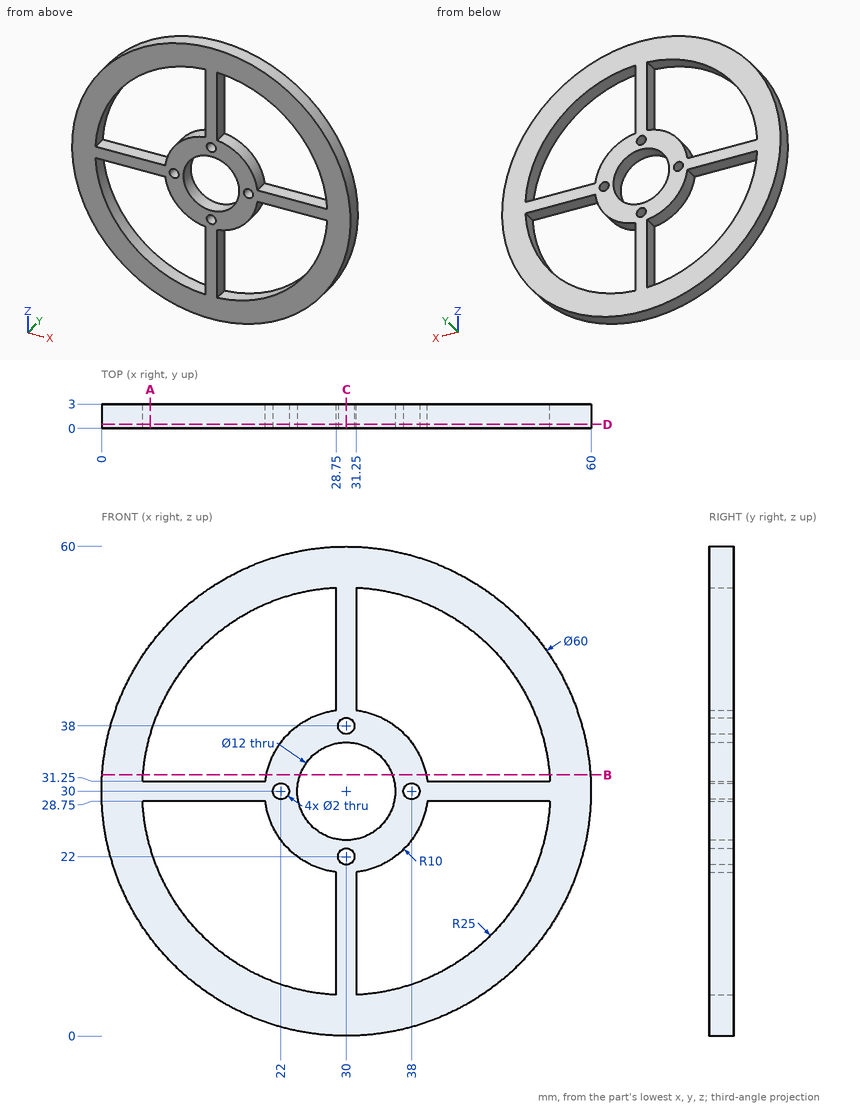
For this review, use the dimensioned drawing (mm, ordinates from the lowest corner) and the shaded views. Give positions to 0.01 mm unless a question says otherwise; leave off trailing zeros. Order: outer loops, then holes, each group sorted by start corner. A loop starts at its lowest first (then second) coordinate and runs counter-clockwise, first axis right, second up.
1) Wall thickness on line 1 (X direction, y = 2.35, z = 30); line 2 (Z direction, x = 36.5, y = 0.6); line 3 (Z direction, x = 49.5, y = 1.95): over which ranges is each line inside the solid? List them lowest first.
2) Take a section at A-A (x = 6). Give the boundary of the cut face in (y, z).
3) Insertion check: pin 1 (1 mm diameter, centred on x = 39, y = 2, fed in from -Z); pin 2 (1.5 mm diameter, centred on x = 13, y = 2, fed in from -Z); pin 3 (1.5 mm diameter, centred on y = 1.5, z = 40.5, fed in from +X). Each pin has a flat end and moves straight along its axis. Give the tip position at first contact, or say it passes through.
4) Take a section at B-B (z = 32). Give the boundary of the cut face in (x, y).
5) Take a section at C-C (x = 30). Give the boundary of the cut face in (y, z).
6) Take a section at D-D (y = 0.5). State how many separate pieces and enclosed holes the cut face has, then the cut area to 3 significant figures.
Derived:
1. line 1: x = 0 to 21, 23 to 24, 36 to 37, 39 to 60
1. line 2: z = 0.71 to 5.86, 22.4 to 37.6, 54.14 to 59.29
1. line 3: z = 7.2 to 14.36, 28.75 to 31.25, 45.64 to 52.8
2. outline: (0, 12) - (3, 12) - (3, 23) - (0, 23) - close; (0, 28.75) - (3, 28.75) - (3, 31.25) - (0, 31.25) - close; (0, 37) - (3, 37) - (3, 48) - (0, 48) - close
3. pin 1: stops at z = 1.23
3. pin 2: stops at z = 4.78
3. pin 3: stops at x = 58.37
4. outline: (0.07, 0) - (5.08, 0) - (5.08, 3) - (0.07, 3) - close; (20.2, 0) - (24.34, 0) - (24.34, 3) - (20.2, 3) - close; (35.66, 0) - (39.8, 0) - (39.8, 3) - (35.66, 3) - close; (54.92, 0) - (59.93, 0) - (59.93, 3) - (54.92, 3) - close
5. outline: (0, 0) - (3, 0) - (3, 21) - (0, 21) - close; (0, 23) - (3, 23) - (3, 24) - (0, 24) - close; (0, 36) - (3, 36) - (3, 37) - (0, 37) - close; (0, 39) - (3, 39) - (3, 60) - (0, 60) - close
6. separate pieces: 1
6. enclosed holes: 9
6. area: 1,200 mm2
